Drawing for the job (mm, zero at the part's lowest x, y, z). Give positions to 0.01 mm unless a question says otherwise; leave off trailing zeros. Loops run counter-clockwise (first coordinate to the right, second up) from the corner with the lowest first, then second, coordinate; pieces in that order, holes last. Notation, with made-up numbers: (54, -38) - (95, -38) arc R27 ccw to (95, -13) - close; hole circle Ø7 at (74, -2). An arc over 180 degrees is marked (long way). Return JSON: item names as keys, results as strings. Group by question number.
1) Mould opens along Z. For the marked faces 1, 2 and 3 say: released by +Z, released by -Z, zero draft, split by the parting line, or undercut.
2) Drill centre lines: probe 1 along Y at (x, z) = (26.5, 10.75) (1 decimal); probe 2 along Z at (x, y) = (14, 11.5) (1 decimal); probe 3 along X at (y, z) = (6.75, 8) (1 decimal). Where is each one in solid material? Low to high. Write a range as from..to.
3) Slice it at A-A (x = 12.5). List the corners of the cut face in (y, z) (1 decimal), and give its area (3 significant figures).
4) Slice it at C-C (z = 2.25). List the corners of the cut face in (x, y).
5) Drop flat-ended pins along their axis: pin 1 (1.5 mm diameter, centred on x = 19, y = 3.5, fed in from -Z); pin 2 (8 mm diameter, centred on x = 4, y = 10.5, fed in from -Z); pin 3 (2 mm diameter, centred on x = 30.5, z = 18.5, fed in from -Y); pin 4 (3 mm diameter, centred on y = 9.5, z = 12, fed in from -X). Give the stop position or say it passes through.
6) Slice it at B-B (y = 16.75). List the corners of the cut face in (x, z) (1 decimal).
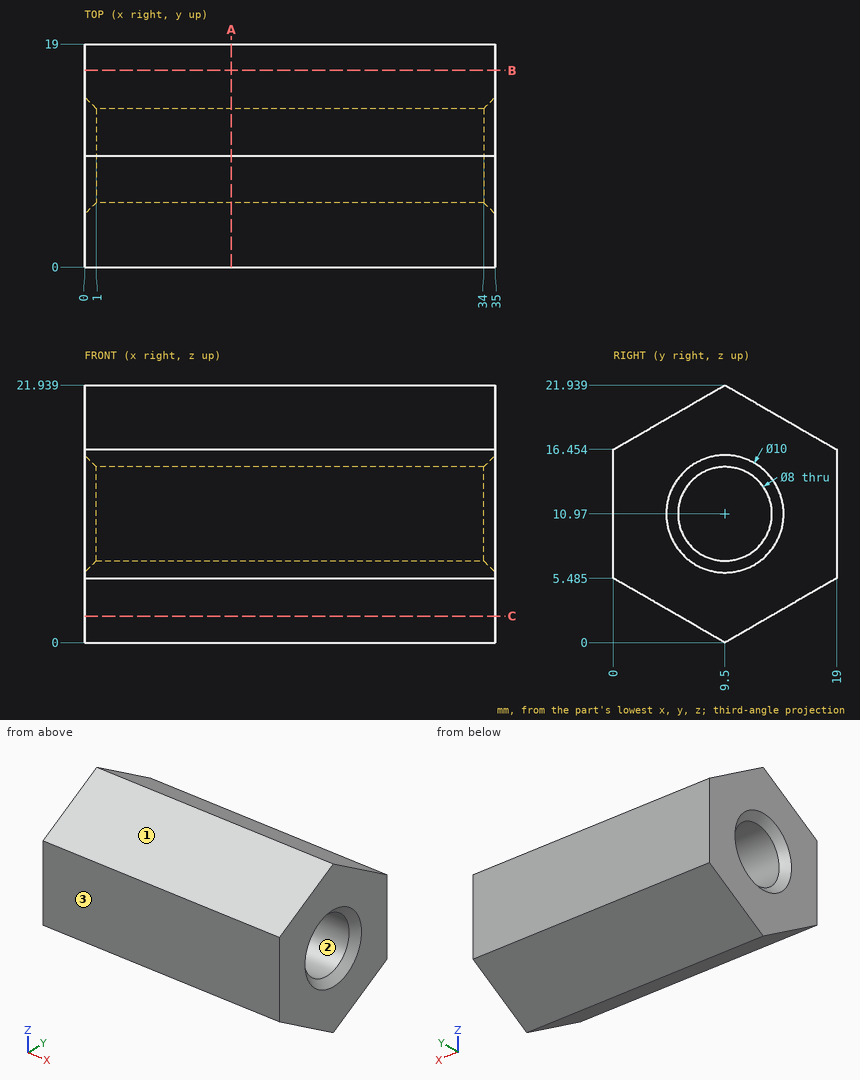
Results:
{
 "1": {"face 1": "released by +Z", "face 2": "undercut", "face 3": "zero draft"},
 "2": {"probe 1": "0..5.5, 13.5..19", "probe 2": "1.2..7.5, 14.4..20.8", "probe 3": "1..34"},
 "3": {"outline": "(0, 5.5) - (9.5, 0) - (19, 5.5) - (19, 16.5) - (9.5, 21.9) - (0, 16.5) - close; hole circle Ø8 at (9.5, 11)", "area": "262 mm2"},
 "4": {"outline": "(0, 5.6) - (35, 5.6) - (35, 13.4) - (0, 13.4) - close"},
 "5": {"pin 1": "z = 3.03", "pin 2": "z = 0", "pin 3": "y = 1.81", "pin 4": "through"},
 "6": {"outline": "(0, 4.2) - (35, 4.2) - (35, 17.8) - (0, 17.8) - close"}
}
